from build123d import *

# Parameters (mm, degrees)
F0_W     = 317.5
F0_H     = 317.5
F1_DEPTH = 6.35
F2_W     = 317.5
F2_H     = 6.35
F3_DEPTH = 38.1
F4_R     = 5.08
F5_R     = 12.7
F6_DEPTH = 25.4


with BuildPart() as f1:
    # F0 (on Top) → F1 (new body)
    with BuildSketch(Plane.XY):
        with Locations((158.75, 172.529013)):
            Rectangle(F0_W, F0_H)
    extrude(amount=F1_DEPTH)

    # F2 (on face) → F3 (join)
    with BuildSketch(Plane(origin=(0, 0, 0), x_dir=(1, 0, 0), z_dir=(0, 0, -1))):
        with Locations((158.75, -16.954013)):
            Rectangle(F2_W, F2_H)
    extrude(amount=F3_DEPTH)

    # F4
    f4_edges = [f1.edges().sort_by_distance(p)[0] for p in [
        (158.75, 13.779013, 6.35),
        (158.75, 20.129013, 0),
    ]]
    fillet(f4_edges, radius=F4_R)

    # F5 (on face) → F6 (cut)
    with BuildSketch(Plane.XY.offset(6.35)):
        with Locations((127, 77.279013)):
            Circle(F5_R)
        with Locations((177.8, 128.079013)):
            Circle(F5_R)
        with Locations((177.8, 216.979013)):
            Circle(F5_R)
        with Locations((127, 280.479013)):
            Circle(F5_R)
    extrude(amount=-F6_DEPTH, mode=Mode.SUBTRACT)


solid = f1.part
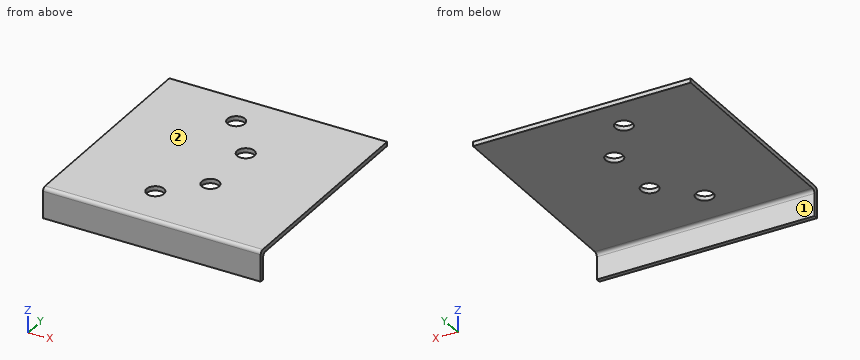
Work out the finished part from the listing and answer in its coordinate system (mm). Face numbers are marked on the shaded views. A direction names the side the tool comes from. Round coordinates to 2 decimals unless told otherwise and drop trailing zeros. Write each loop counter-clockwise with the first axis right and the second up, starting at its lowest first coordinate (ties: lowest second). Pieces come first, ordered by that corner, then holes. Notation, with made-up numbers: (3, 16.25) -> (38, 16.25) arc R23 ccw to (38, 28.25) -> close; hole circle Ø9 at (85.5, 27). An arc over 180 degrees is marked (long way). Write each question's results on one line, items separated by ' | '.
Item 1: A cutting plane is placed at C-C, the plane x = 283. Determine the outline of the cut face in (y, z).
Result set:
outline: (13.78, -38.1) -> (20.13, -38.1) -> (20.13, -5.08) arc R5.08 cw to (25.21, 0) -> (331.28, 0) -> (331.28, 6.35) -> (18.86, 6.35) arc R5.08 ccw to (13.78, 1.27) -> close
Item 2: Find the intervals of material crossed by line 1 along Y through (x, z) = (127, 2); line 2 along Y through (x, z) = (177, 4); line 3 along Z through (x, y) = (115, 188), in increasing order. Write a range as [from, to].
Result set:
line 1: [13.83, 64.58], [89.98, 267.78], [293.18, 331.28] | line 2: [14.57, 115.4], [140.75, 204.3], [229.65, 331.28] | line 3: [0, 6.35]
Item 3: A cutting plane is placed at A-A, the plane x = 127. Determine the outline of the cut face in (y, z).
Result set:
outline: (13.78, -38.1) -> (20.13, -38.1) -> (20.13, -5.08) arc R5.08 cw to (25.21, 0) -> (64.58, 0) -> (64.58, 6.35) -> (18.86, 6.35) arc R5.08 ccw to (13.78, 1.27) -> close; (89.98, 0) -> (267.78, 0) -> (267.78, 6.35) -> (89.98, 6.35) -> close; (293.18, 0) -> (331.28, 0) -> (331.28, 6.35) -> (293.18, 6.35) -> close
Item 4: A cutting plane is placed at B-B, the plane y = 121.5. Determine the outline of the cut face in (x, z), plus the area to 3 significant figures.
Result set:
outline: (0, 0) -> (166.94, 0) -> (166.94, 6.35) -> (0, 6.35) -> close; (188.66, 0) -> (317.5, 0) -> (317.5, 6.35) -> (188.66, 6.35) -> close | area: 1,880 mm^2
Item 5: A cutting plane is placed at D-D, the plane z = -9. Determine the outline of the cut face in (x, y).
Result set:
outline: (0, 13.78) -> (317.5, 13.78) -> (317.5, 20.13) -> (0, 20.13) -> close
Item 6: Flat-ended cylindrical pins translate along their axes: P1, Ø1.5, axis at x = 245, z = -22.5, coming from the +Y side; P2, Ø6, axis at x = 260, y = 272.5, coming from the -Z side. Find the tip coordinate at first contact, or state that the pin passes through.
Result set:
P1: y = 20.13 | P2: z = 0
Item 7: Which of the six approach directions +Z, -Z, +X, -X, +Y, -Y give full straight-line access (tool end or side, diameter ignored) to the marked faces 1 and 2?
Result set:
face 1: -Z, +X, -X, +Y | face 2: +Z, +X, -X, +Y, -Y
